Verification items for the finished model (mm, model axes). A direction names the side the tool comes from. Give positions to 0.01 mm unless a question says otherwise; leave off trailing zeros. Order: outer loops, then holes, each group sorted by start corner. A loop starts at its lowest first (then second) coordinate and runs counter-clockwise, first axis right, second up. Notation, with made-up numbers: (13, 40) - (47, 40) arc R26 ccw to (47, 69) - close; hole circle Ø10 at (-7.5, 23). An arc over 180 degrees is marked (long way). Answer as a JSON object with one key per item and string values. Group by question number.
(1) Section check A-A (x = 0). Record the boundary of the cut face in (y, z) (3 decimals).
(2) Section check D-D (y = -32). Record the boundary of the cut face in (x, z) (3 decimals).
(3) Thickness scan on line 1 (Y direction, x = 34, z = 5.75); line 2 (Y direction, x = 21, z = 2.3) (3 decimals); line 3 (Y direction, x = 0, z = 2.5) (3 decimals). Record the ranges inside material, lowest first.
(4) Depth check by flat-ended pin: pin 1 Ø3.5 at (x, y) = (29, 21) entering from +Z; pin 2 Ø5.5 at (x, y) = (0, 21) entering from -Z. Enter the tip coordinate at first touch or a pass-through.
(5) Access from +Z, -Z, +X, -X, +Y, -Y to the whole of each face (thin tool, end or side, straight path). Record for faces 4 (the face through (-32.869, 23.966, 2.465)), 5 (the face through (30.548, 19.581, 7.535)).
(6) Section check C-C (x = -21). Record the boundary of the cut face in (y, z) (3 decimals).
(7) Mould release check, pull along Y, two halves, no side actions. Record for faces 1 (the face through (-1, -42, 5)), 2 (the face through (18.997, -10.631, 7.535)), 3 (the face through (-1, 1, 10)): +Y half, -Y half, draft (parallel to the pull), parting line (faces both ways), or undercut.
(8) Section check B-B (z = 3.5). Count the separate pieces of the cut face and the enclosed holes in it, then the cut area to 3 significant figures.
```python
from build123d import *

# Parameters (mm, degrees)
F0_W           = 84
F0_H           = 84
F1_DEPTH       = 10
F3_D           = 4.2
F5_D           = 4.2
F5_CBORE_D     = 9.75
F5_CBORE_DEPTH = 5


# Not quite as in the source:
# - a feature names something its author has since deleted; it is built from what else it names


with BuildPart() as f1:
    # F0 (on Top) → F1 (new body)
    with BuildSketch(Plane.XY):
        Rectangle(F0_W, F0_H)
    extrude(amount=F1_DEPTH)

    # F3 (through all)
    with Locations(Plane.XY.offset(10)):
        with Locations((-34, 36.25), (-8, 36.25), (8, 36.25), (34, 36.25), (34, 5.75), (8, 5.75), (-8, 5.75), (-34, 5.75), (0, -11), (0, -31)):
            Hole(F3_D / 2)

    # F5 (through all)
    with Locations(Plane(origin=(0, 0, 0), x_dir=(1, 0, 0), z_dir=(0, 0, -1))):
        with Locations((29, -21), (0, -21), (-29, -21), (21, 10), (21, 32), (-21, 32), (-21, 10)):
            CounterBoreHole(F5_D / 2, F5_CBORE_D / 2, F5_CBORE_DEPTH)


solid = f1.part
```
Solutions:
{
 "1": {"outline": "(-42, 0) - (-33.1, 0) - (-33.1, 10) - (-42, 10) - close; (-28.9, 0) - (-13.1, 0) - (-13.1, 10) - (-28.9, 10) - close; (-8.9, 0) - (16.125, 0) - (16.125, 5) - (18.9, 5) - (18.9, 10) - (-8.9, 10) - close; (23.1, 5) - (25.875, 5) - (25.875, 0) - (42, 0) - (42, 10) - (23.1, 10) - close"},
 "2": {"outline": "(-42, 0) - (-25.875, 0) - (-25.875, 5) - (-23.1, 5) - (-23.1, 10) - (-42, 10) - close; (-18.9, 5) - (-16.125, 5) - (-16.125, 0) - (-1.847, 0) - (-1.847, 10) - (-18.9, 10) - close; (1.847, 0) - (16.125, 0) - (16.125, 5) - (18.9, 5) - (18.9, 10) - (1.847, 10) - close; (23.1, 5) - (25.875, 5) - (25.875, 0) - (42, 0) - (42, 10) - (23.1, 10) - close"},
 "3": {"line 1": "y = -42 to 3.65, 7.85 to 34.15, 38.35 to 42", "line 2": "y = -42 to -36.875, -27.125 to -14.875, -5.125 to 42", "line 3": "y = -42 to -33.1, -28.9 to -13.1, -8.9 to 16.125, 25.875 to 42"},
 "4": {"pin 1": "passes through", "pin 2": "stops at z = 5"},
 "5": {"face 4": "-Z", "face 5": "+Z, -Z"},
 "6": {"outline": "(-42, 0) - (-36.875, 0) - (-36.875, 5) - (-34.1, 5) - (-34.1, 10) - (-42, 10) - close; (-29.9, 5) - (-27.125, 5) - (-27.125, 0) - (-14.875, 0) - (-14.875, 5) - (-12.1, 5) - (-12.1, 10) - (-29.9, 10) - close; (-7.9, 5) - (-5.125, 5) - (-5.125, 0) - (42, 0) - (42, 10) - (-7.9, 10) - close"},
 "7": {"face 1": "-Y half", "face 2": "undercut", "face 3": "draft"},
 "8": {"separate pieces": "1", "enclosed holes": "17", "area": "6,390 mm2"}
}
